```python
from build123d import *

# Parameters (mm, degrees)
SKETCH1_R                = 75
BOSS_EXTRUDE1_DEPTH      = 30
SKETCH2_W                = 16.050334996
SKETCH2_H                = 27
BOSS_EXTRUDE3_DEPTH      = 30
SKETCH3_R                = 1.5
CUT_EXTRUDE3_DEPTH       = 57.805954881
CUT_EXTRUDE3_DEPTH_BACK  = 94.194045119
SKETCH4_R                = 1.5
CUT_EXTRUDE4_DEPTH       = 148.645950403
SKETCH6_R                = 1.5
CUT_EXTRUDE5_DEPTH       = 148.645950403
SKETCH7_W                = 16.050693915
SKETCH7_H                = 21
CUT_EXTRUDE6_DEPTH       = 24
CUT_EXTRUDE7_DEPTH       = 24
CUT_EXTRUDE8_DEPTH       = 24
FILLET4_R                = 3
CUT_EXTRUDE9_DEPTH       = 25
CUT_EXTRUDE9_DEPTH_BACK  = 37
CUT_EXTRUDE10_DEPTH      = 25
CUT_EXTRUDE10_DEPTH_BACK = 37
SKETCH12_W               = 95
SKETCH12_H               = 21
CUT_EXTRUDE11_DEPTH      = 25
CUT_EXTRUDE11_DEPTH_BACK = 37
FILLET5_R                = 5
FILLET6_R                = 3
FILLET7_R                = 3


with BuildPart() as part:
    # Sketch1 → Boss-Extrude1 (new body)
    with BuildSketch(Plane(origin=(0, 0, 0), x_dir=(1, 0, 0), z_dir=(0, 1, 0))):
        Circle(SKETCH1_R)
    extrude(amount=BOSS_EXTRUDE1_DEPTH)

    # Sketch2 → Boss-Extrude3 (add)
    with BuildSketch(Plane(origin=(0, 30, 0), x_dir=(1, 0, 0), z_dir=(0, 1, 0))):
        Polygon((3.333824547, 30.61373674), (26.716510449, 44.11373674), (18.691342951, 58.013734586), (-4.691342951, 44.513734586), align=None)
        with Locations((32.870528946, -31.694045119)):
            Rectangle(SKETCH2_W, SKETCH2_H)
        Polygon((-59.587039395, -12.819689466), (-36.204353493, -26.319689466), (-28.179185995, -12.419691621), (-51.561871897, 1.080308379), align=None)
    extrude(amount=BOSS_EXTRUDE3_DEPTH)

    # Sketch3 → Cut-Extrude3 (cut, two sides)
    with BuildSketch(Plane(origin=(24.845361448, 30, 18.194045119), x_dir=(1, 0, 0), z_dir=(0, 0, 1))) as cut_extrude3_sk:
        with Locations((8.025167498, 25)):
            Circle(SKETCH3_R)
    extrude(amount=CUT_EXTRUDE3_DEPTH, mode=Mode.SUBTRACT)
    extrude(cut_extrude3_sk.sketch, amount=-CUT_EXTRUDE3_DEPTH_BACK, mode=Mode.SUBTRACT)

    # Sketch4 → Cut-Extrude4 (cut, through all)
    with BuildSketch(Plane(origin=(-39.139191173, 0, -22.59702256), x_dir=(-0.5, 0, 0.866025404), z_dir=(-0.866025404, 0, -0.5))):
        with Locations((32.870528946, 55)):
            Circle(SKETCH4_R)
    extrude(amount=-CUT_EXTRUDE4_DEPTH, mode=Mode.SUBTRACT)

    # Sketch6 → Cut-Extrude5 (cut, through all)
    with BuildSketch(Plane(origin=(39.139191173, 0, -22.59702256), x_dir=(-0.5, 0, -0.866025404), z_dir=(0.866025404, 0, -0.5))):
        with Locations((32.870528946, 55)):
            Circle(SKETCH6_R)
    extrude(amount=-CUT_EXTRUDE5_DEPTH, mode=Mode.SUBTRACT)

    # Sketch7 → Cut-Extrude6 (cut)
    with BuildSketch(Plane(origin=(0, 60, 0), x_dir=(1, 0, 0), z_dir=(0, 1, 0))):
        with Locations((32.870349487, -31.694045119)):
            Rectangle(SKETCH7_W, SKETCH7_H)
    extrude(amount=-CUT_EXTRUDE6_DEPTH, mode=Mode.SUBTRACT)

    # Sketch8 → Cut-Extrude7 (cut)
    with BuildSketch(Plane(origin=(0, 60, 0), x_dir=(1, 0, 0), z_dir=(0, 1, 0))):
        Polygon((-30.777262206, -10.919691621), (-48.963795686, -0.419691621), (-56.988963184, -14.319689466), (-38.802429704, -24.819689466), align=None)
    extrude(amount=-CUT_EXTRUDE7_DEPTH, mode=Mode.SUBTRACT)

    # Sketch9 → Cut-Extrude8 (cut)
    with BuildSketch(Plane(origin=(0, 60, 0), x_dir=(1, 0, 0), z_dir=(0, 1, 0))):
        Polygon((16.09326674, 56.513734586), (24.118434238, 42.61373674), (5.931900758, 32.11373674), (-2.09326674, 46.013734586), align=None)
    extrude(amount=-CUT_EXTRUDE8_DEPTH, mode=Mode.SUBTRACT)

    # Fillet4
    fillet4_edges = [part.edges().sort_by_distance(p)[0] for p in [
        (24.845361448, 30, 31.694045119),
        (32.870528946, 30, 45.194045119),
        (40.895696444, 30, 31.694045119),
        (32.870528946, 30, 18.194045119),
        (22.7039267, 30, -51.063735663),
        (7, 30, -51.263734586),
        (-0.678759202, 30, -37.563735663),
        (15.025167498, 30, -37.36373674),
        (-32.191769744, 30, 19.369690543),
        (-39.870528946, 30, 5.669691621),
        (-55.574455646, 30, 5.869690543),
        (-47.895696444, 30, 19.569689466),
    ]]
    fillet(fillet4_edges, radius=FILLET4_R)

    # Sketch10 → Cut-Extrude9 (cut, two sides)
    with BuildSketch(Plane(origin=(0, 36, 0), x_dir=(1, 0, 0), z_dir=(0, 1, 0))) as cut_extrude9_sk:
        Polygon((-25.01267474, 41.064866756), (-6.82614126, 30.564866756), (-54.32614126, -51.707546603), (-72.51267474, -41.207546603), align=None)
    extrude(amount=CUT_EXTRUDE9_DEPTH, mode=Mode.SUBTRACT)
    extrude(cut_extrude9_sk.sketch, amount=-CUT_EXTRUDE9_DEPTH_BACK, mode=Mode.SUBTRACT)

    # Sketch11 → Cut-Extrude10 (cut, two sides)
    with BuildSketch(Plane(origin=(0, 36, 0), x_dir=(1, 0, 0), z_dir=(0, 1, 0))) as cut_extrude10_sk:
        Polygon((-17.616978296, 72.901591723), (0.569555184, 83.401591723), (48.069555184, 1.129178363), (29.883021704, -9.370821637), align=None)
    extrude(amount=CUT_EXTRUDE10_DEPTH, mode=Mode.SUBTRACT)
    extrude(cut_extrude10_sk.sketch, amount=-CUT_EXTRUDE10_DEPTH_BACK, mode=Mode.SUBTRACT)

    # Sketch12 → Cut-Extrude11 (cut, two sides)
    with BuildSketch(Plane(origin=(0, 36, 0), x_dir=(1, 0, 0), z_dir=(0, 1, 0))) as cut_extrude11_sk:
        with Locations((24.443119556, -31.694045119)):
            Rectangle(SKETCH12_W, SKETCH12_H)
    extrude(amount=CUT_EXTRUDE11_DEPTH, mode=Mode.SUBTRACT)
    extrude(cut_extrude11_sk.sketch, amount=-CUT_EXTRUDE11_DEPTH_BACK, mode=Mode.SUBTRACT)

    # Fillet5
    fillet5_edges = [part.edges().sort_by_distance(p)[0] for p in [
        (-67.543786445, 15, 32.60117962),
        (-54.32614126, 15, 51.707546603),
        (5.538443478, 15, -74.79522474),
        (-17.616978296, 15, -72.901591723),
        (62.005342967, 15, 42.194045119),
        (71.943119556, 15, 21.194045119),
    ]]
    fillet(fillet5_edges, radius=FILLET5_R)

    # Fillet6
    fillet6_edges = [part.edges().sort_by_distance(p)[0] for p in [
        (-25.01267474, 15, -41.064866756),
        (-6.82614126, 15, -30.564866756),
        (29.883021704, 15, 9.370821637),
        (48.069555184, 15, -1.129178363),
        (-23.056880444, 15, 42.194045119),
        (-23.056880444, 15, 21.194045119),
    ]]
    fillet(fillet6_edges, radius=FILLET6_R)

    # Fillet7
    fillet7_edges = [part.edges().sort_by_distance(p)[0] for p in [
        (-3.392304845, 60, -45.263734586),
        (25.417472343, 60, -43.36373674),
        (24.845361448, 60, 19.694045119),
        (40.895696444, 60, 43.694045119),
        (17.392304845, 60, -57.263734586),
        (4.632862653, 60, -31.36373674),
        (24.845361448, 60, 43.694045119),
        (40.895696444, 60, 19.694045119),
        (-50.262833792, 60, -0.330308379),
        (-37.503391599, 60, 25.569689466),
        (-29.478224101, 60, 11.669691621),
        (-58.28800129, 60, 13.569689466),
    ]]
    fillet(fillet7_edges, radius=FILLET7_R)


solid = part.part
```
Here's how the part is built. I have some questions about the finished solid (model axes, mm). A direction names the side the tool comes from. Round coordinates to 2 decimals unless told otherwise and drop trailing zeros. Write each loop counter-clockwise with the first axis right and the second up, starting at its lowest first coordinate (ties: lowest second). Pieces come first, ordered by that corner, then holes.
Q1. If we section it at B-B on z = 60: Write out the boundary of the cut face in (x, y), plus the area to 3 significant figures.
Q2. Please list where these lines run through material, in increasing order: probe 1 along Z at (x, y) = (33, 9); probe 2 along Z at (x, y) = (26.5, 13.5); probe 3 along X at (y, z) = (55, 19).
Q3. If we mould it in two halves opening along X, with no side actions, what happens to faces 1 (the cylindrical face through (-24.723, 14.79, -39.856)), 2 (the flat face through (-1, 0, 0)), 3 (the cylindrical face through (-28.14, 30.52, 10.93))? For each: +X half, -X half, draft (parallel to the pull), parting line (faces both ways), or undercut.
Q4. Will these pins go through, and if not, where does the flat tip stop? P1, Ø5, axis at x = 42, z = -40, coming from the +Y side; P2, Ø1, axis at y = 16, z = -35, coming from the -X side; P3, Ø0.9, axis at y = 47, z = 43, coming from the +X side; P4, Ø1.5, axis at x = 54, z = 22.5, coming from the +Y side.
Q5. If we section it at A-A on y = 4.5: Write out the boundary of the cut face in (x, z), plus the area to 3 significant figures.
Q6. Which directions (+Z, -Z, +X, -X, +Y, -Y) give clear straight access to the entire face, cutting with the end or side of a thin tool? Please do faces 4 (the cylindrical face through (-8.035, 14.79, -30.275)), 5 (the flat face through (-32.25, 46.31, 19.47)), 6 (the cylindrical face through (26.829, 30.524, -42.67)).
Answer below:
1. outline: (-45, 0) - (45, 0) - (45, 30) - (-45, 30) - close
1. area: 2,700 mm2
2. probe 1: z = -67.35 to -27.23, 7.57 to 21.19, 42.19 to 67.35
2. probe 2: z = -70.16 to -38.49, 3.51 to 21.19, 42.19 to 70.16
2. probe 3: x = 24.85 to 31.37, 34.37 to 40.9
3. face 1: undercut
3. face 2: draft
3. face 3: +X half
4. P1: stops at y = 30
4. P2: stops at x = -66.59
4. P3: stops at x = 40.9
4. P4: passes through
5. outline: (-71.49, 22.69) arc R75 ccw to (-21.46, -71.87) arc R5 ccw to (-15.7, -69.57) - (28.38, 6.77) arc R3 cw to (32.48, 7.87) - (45.47, 0.37) arc R3 cw to (46.57, -3.73) - (10.69, -65.87) arc R5 ccw to (16.1, -73.25) arc R75 ccw to (72.97, 17.35) arc R5 ccw to (68.1, 21.19) - (-20.06, 21.19) arc R3 cw to (-23.06, 24.19) - (-23.06, 39.19) arc R3 cw to (-20.06, 42.19) - (51.7, 42.19) arc R5 ccw to (55.39, 50.57) arc R75 ccw to (-51.51, 54.51) arc R5 ccw to (-52.41, 48.38) - (-8.33, -27.97) arc R3 cw to (-9.42, -32.06) - (-22.41, -39.56) arc R3 cw to (-26.51, -38.47) - (-62.39, 23.68) arc R5 ccw to start
5. area: 11,900 mm2
6. face 4: +Y, -Y
6. face 5: +Z, +Y
6. face 6: +X, +Y
